Geometry check sheet. Reference: the model listing, model coordinates, mm. A direction names the side the tool comes from. Round coordinates to 2 decimals unless told otherwise and drop trailing zeros. Order: outer loops, then holes, each group sorted by start corner. A loop starts at its lowest first (then second) coordinate and runs counter-clockwise, first axis right, second up.
(1) Cross-section at C-C on z = -3. Enter the section's corners in (x, y), and give its area (3 significant figures).
(2) Gauge pin test, flat ends, axial feed: P1, Ø7, axis at x = 0, z = -9.01, coming from the -Y side; P2, Ø4, axis at x = -11, z = -22, coming from the +Y side; P3, Ø2, axis at y = 20, z = -34.5, coming from the -X side; P4, Ø24, axis at x = 5, y = 5, coming from the -Z side. Record the tip position at first contact, or that the pin passes through.
(3) Draft check along X on faces 4 (the face through (-31.24, -6.94, -36.58)), 5 (the face through (-7, 15, 22.985)), 6 (the face through (-0.39, 22.76, -11.99)). Enter one of: pulls with the +X half, pulls with the -X half, needs draft (parallel to the pull), parting line crosses it, or undercut.
(4) Thickness scan on L1, parallel to Z at x = 0, y = 23.5; L2, parallel to Z at x = 0, y = 20; L3, parallel to Y at x = 0, z = 4. Record the ranges inside material, lowest first.
(5) Cross-section at D-D on x = 14. Enter the section's corners in (y, z).
(6) Cross-section at B-B on x = 0. Count the separate pieces of the cut face and the enclosed holes in it, and give its area (3 significant figures).
(7) Set-up check for faces 1 (the face through (-0.52, 25.76, -12.98)), 2 (the face through (3, 30, -10)), 3 (the face through (-8.43, 20.32, -9.21)): record each of +Z, -Z, +X, -X, +Y, -Y from which the full face is reachable in a straight line by a thin tool's end or side.
(8) Cross-section at A-A on y = 0. Enter the section's corners in (x, z).
from build123d import *

# Parameters (mm, degrees)
BOSS_EXTRUDE1_START     = 22
SKETCH3_R               = 4
BOSS_EXTRUDE1_DEPTH     = 8
BOSS_EXTRUDE2_START     = -2e-06
SKETCH4_R               = 4
BOSS_EXTRUDE2_DEPTH     = 0.366694
SKETCH2_R               = 3
CUT_EXTRUDE2_DEPTH      = 33
CUT_EXTRUDE2_DEPTH_BACK = 33


with BuildPart() as part:
    # Sketch1 → Revolve1 (revolve)
    with BuildSketch(Plane(origin=(0, 0, 0), x_dir=(0, 0, -1), z_dir=(1, 0, 0))):
        Polygon((-22.985422917, 16), (-22.985422917, 32), (-13.985422917, 32), (-13.985422917, 24), (-4.985422917, 24), (-4.985422917, 22), (23.014577083, 22), (23.014577083, 27.022421525), (32.014577083, 27.022421525), (32.014577083, 32), (41.014577083, 32), (41.014577083, 16), align=None)
    revolve(axis=Axis((0, 0, 0), (0, 0, -1)))



with BuildPart() as body_2:
    # Sketch3 → Boss-Extrude1 (new body)
    with BuildSketch(Plane(origin=(0, 0, 0), x_dir=(1, 0, 0), z_dir=(0, 1, 0)).offset(BOSS_EXTRUDE1_START)):
        with Locations((0, 9.014577083)):
            Circle(SKETCH3_R)
    extrude(amount=BOSS_EXTRUDE1_DEPTH)


with BuildPart() as part_1:
    add(part.part)

    add(body_2.part)  # Boss-Extrude2 merges body 2
    # Sketch4 → Boss-Extrude2 (add)
    with BuildSketch(Plane.XZ.offset(-22).offset(BOSS_EXTRUDE2_START)):
        with Locations((0, -9.014577083)):
            Circle(SKETCH4_R)
    extrude(amount=BOSS_EXTRUDE2_DEPTH)

    # Sketch2 → Cut-Extrude2 (cut, two sides)
    with BuildSketch(Plane(origin=(0, 0, 0), x_dir=(1, 0, 0), z_dir=(0, 1, 0))) as cut_extrude2_sk:
        with Locations((0, 9.014577083)):
            Circle(SKETCH2_R)
    extrude(amount=CUT_EXTRUDE2_DEPTH, mode=Mode.SUBTRACT)
    extrude(cut_extrude2_sk.sketch, amount=-CUT_EXTRUDE2_DEPTH_BACK, mode=Mode.SUBTRACT)


solid = part_1.part
Found:
1. outline: circle Ø44 at (0, 0); hole circle Ø32 at (0, 0)
1. area: 716 mm2
2. P1: stops at y = -22
2. P2: stops at y = 25.38
2. P3: stops at x = -25.75
2. P4: stops at z = -41.01
3. face 4: parting line crosses it
3. face 5: needs draft
3. face 6: undercut
4. L1: z = -41.01 to -23.01, -13.01 to -12.01, -6.01 to -5.01, 4.99 to 22.99
4. L2: z = -41.01 to -12.01, -6.01 to 22.99
4. L3: y = -22 to -16, 16 to 22
5. outline: (-28.77, -41.01) - (-7.75, -41.01) - (-7.75, 22.99) - (-28.77, 22.99) - (-28.77, 13.99) - (-19.49, 13.99) - (-19.49, 4.99) - (-16.97, 4.99) - (-16.97, -23.01) - (-23.11, -23.01) - (-23.11, -32.01) - (-28.77, -32.01) - close; (7.75, -41.01) - (28.77, -41.01) - (28.77, -32.01) - (23.11, -32.01) - (23.11, -23.01) - (16.97, -23.01) - (16.97, 4.99) - (19.49, 4.99) - (19.49, 13.99) - (28.77, 13.99) - (28.77, 22.99) - (7.75, 22.99) - close
6. separate pieces: 4
6. enclosed holes: 0
6. area: 1,200 mm2
7. face 1: +Y
7. face 2: +X, -X, +Y
7. face 3: none
8. outline: (-32, -41.01) - (-16, -41.01) - (-16, 22.99) - (-32, 22.99) - (-32, 13.99) - (-24, 13.99) - (-24, 4.99) - (-22, 4.99) - (-22, -23.01) - (-27.02, -23.01) - (-27.02, -32.01) - (-32, -32.01) - close; (16, -41.01) - (32, -41.01) - (32, -32.01) - (27.02, -32.01) - (27.02, -23.01) - (22, -23.01) - (22, 4.99) - (24, 4.99) - (24, 13.99) - (32, 13.99) - (32, 22.99) - (16, 22.99) - close
